CAD build for the part. Positions are in the model's coordinates, mm. Give positions to 0.01 mm unless a question says otherwise; leave off trailing zeros. Loops run counter-clockwise (first coordinate to the right, second up) from the corner with the lowest first, then second, coordinate; pieces in that order, holes last. Notation, with made-up numbers: M 42,-20 L 88,-20 A23 ccw 88,9 Z; hole C -27,-25.5 d1. An arc over 180 degrees is marked long. Answer as CSV lines item,"result".
```python
from build123d import *

# Parameters (mm, degrees)
EXTRUDE_1_DEPTH          = 2
CUT_EXTRUDE_1_DEPTH      = 2
PATTERN_START            = -2
PATTERN_LINEAR_1_DEPTH   = 2
PATTERN_CIRCULAR_2_COUNT = 5


# Read off the part's stored shape, not the designer's step: Линейный массив1
with BuildPart() as part:
    # Эскиз1 → Бобышка-Вытянуть1 (new body)
    with BuildSketch(Plane.XY):
        with BuildLine():
            Line((-21.160269083, 29.124611797), (0, 0))
            Line((0, 0), (21.160269083, 29.124611797))
            ThreePointArc((21.160269083, 29.124611797), (0, 36), (-21.160269083, 29.124611797))
        make_face()
    extrude_1 = extrude(amount=-EXTRUDE_1_DEPTH)

    # Эскиз3 → Вырез-Вытянуть1 (cut)
    with BuildSketch(Plane(origin=(0, 0, -2), x_dir=(-1, 0, 0), z_dir=(0, 0, -1))):
        with BuildLine():
            ThreePointArc((2.821419138, 8.689986144), (0, 9.136534635), (-2.821419138, 8.689986144))
            ThreePointArc((-2.821419138, 8.689986144), (-3.624317507, 7.115072112), (-2.049403475, 6.312173743))
            ThreePointArc((-2.049403475, 6.312173743), (0, 6.636534635), (2.049403475, 6.312173743))
            ThreePointArc((2.049403475, 6.312173743), (3.624317507, 7.115072112), (2.821419138, 8.689986144))
        make_face()
    cut_extrude_1 = extrude(amount=-CUT_EXTRUDE_1_DEPTH, mode=Mode.SUBTRACT)

    # Линейный массив1 outline → Линейный массив1 (cut)
    with BuildSketch(Plane.XY.offset(PATTERN_START)):
        with BuildLine():
            ThreePointArc((-5.868267845, 12.702937061), (-6.478815917, 11.043952114), (-4.81983097, 10.433404043))
            ThreePointArc((-4.81983097, 10.433404043), (0, 11.492897394), (4.81983097, 10.433404043))
            ThreePointArc((4.81983097, 10.433404043), (6.478815917, 11.043952114), (5.868267845, 12.702937061))
            ThreePointArc((5.868267845, 12.702937061), (0, 13.992897394), (-5.868267845, 12.702937061))
        make_face()
        with BuildLine():
            ThreePointArc((-14.786044108, 24.78794491), (-15.219207741, 23.074069399), (-13.50533223, 22.640905767))
            ThreePointArc((-13.50533223, 22.640905767), (0, 26.362940135), (13.50533223, 22.640905767))
            ThreePointArc((13.50533223, 22.640905767), (15.219207741, 23.074069399), (14.786044108, 24.78794491))
            ThreePointArc((14.786044108, 24.78794491), (0, 28.862940135), (-14.786044108, 24.78794491))
        make_face()
        with BuildLine():
            ThreePointArc((-17.738574213, 28.824927916), (-18.148018532, 27.10523162), (-16.428322236, 26.695787302))
            ThreePointArc((-16.428322236, 26.695787302), (0, 31.345730668), (16.428322236, 26.695787302))
            ThreePointArc((16.428322236, 26.695787302), (18.148018532, 27.10523162), (17.738574213, 28.824927916))
            ThreePointArc((17.738574213, 28.824927916), (0, 33.845730668), (-17.738574213, 28.824927916))
        make_face()
        with BuildLine():
            ThreePointArc((-8.858865357, 16.724555129), (-9.378370621, 15.034846787), (-7.688662279, 14.515341523))
            ThreePointArc((-7.688662279, 14.515341523), (0, 16.4259145), (7.688662279, 14.515341523))
            ThreePointArc((7.688662279, 14.515341523), (9.378370621, 15.034846787), (8.858865357, 16.724555129))
            ThreePointArc((8.858865357, 16.724555129), (0, 18.9259145), (-8.858865357, 16.724555129))
        make_face()
        with BuildLine():
            ThreePointArc((-11.827697591, 20.75389585), (-12.294790819, 19.04895482), (-10.589849789, 18.581861592))
            ThreePointArc((-10.589849789, 18.581861592), (0, 21.387624898), (10.589849789, 18.581861592))
            ThreePointArc((10.589849789, 18.581861592), (12.294790819, 19.04895482), (11.827697591, 20.75389585))
            ThreePointArc((11.827697591, 20.75389585), (0, 23.887624898), (-11.827697591, 20.75389585))
        make_face()
    pattern_linear_1 = extrude(amount=PATTERN_LINEAR_1_DEPTH, mode=Mode.SUBTRACT)

    # Круговой массив2: Бобышка-Вытянуть1, Вырез-Вытянуть1, Линейный массив1 ×5 about axis
    pattern_circular_2_axis = Axis((0, 0, 0), (0, 0, 1))
    add([extrude_1.rotate(pattern_circular_2_axis, i * 360 / PATTERN_CIRCULAR_2_COUNT) for i in range(1, PATTERN_CIRCULAR_2_COUNT)])
    add([cut_extrude_1.rotate(pattern_circular_2_axis, i * 360 / PATTERN_CIRCULAR_2_COUNT) for i in range(1, PATTERN_CIRCULAR_2_COUNT)], mode=Mode.SUBTRACT)
    add([pattern_linear_1.rotate(pattern_circular_2_axis, i * 360 / PATTERN_CIRCULAR_2_COUNT) for i in range(1, PATTERN_CIRCULAR_2_COUNT)], mode=Mode.SUBTRACT)


solid = part.part
```
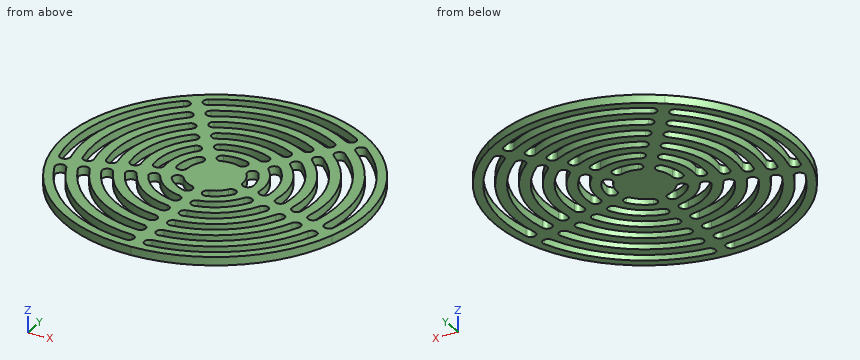
Q1. Cut at A-A (y = 28). Write the cut outline in (x, z), and give its area (3 significant figures).
Solution:
outline,"M -22.63,-2 L -18.31,-2 L -18.31,0 L -22.63,0 Z; M -14.09,-2 L -7,-2 L -7,0 L -14.09,0 Z; M 7,-2 L 14.09,-2 L 14.09,0 L 7,0 Z; M 18.31,-2 L 22.63,-2 L 22.63,0 L 18.31,0 Z"
area,"45.6 mm²"
Q2. Wall check: line 1 (Y direction, x = -22, z = -1.55); line 2 (Y direction, x = -19, z = -0.7); line 3 (Y direction, x = -29, z = -1.65). Give the ranges that are in metal, low to high. Write a range as [from, to].
Solution:
line 1,"y = [-28.5, -25.72], [-22.33, -18.68], [-14.53, -5.82], [9.31, 14.53], [18.68, 22.33], [25.72, 28.5]"
line 2,"y = [-30.58, -28.01], [-24.93, -21.73], [-18.28, -14.48], [-9.82, 9.82], [14.48, 18.28], [21.73, 30.58]"
line 3,"y = [-21.33, -17.45], [-11.9, 11.9], [17.45, 21.33]"
Q3. Cut at B-B (y = -27.5). Write the cut outline in (x, z), and give its area (3 significant figures).
Solution:
outline,"M -23.23,-2 L -19.73,-2 L -19.73,0 L -23.23,0 Z; M -15.04,-2 L -8.76,-2 L -8.76,0 L -15.04,0 Z; M -1.24,-2 L 1.24,-2 L 1.24,0 L -1.24,0 Z; M 8.76,-2 L 15.04,-2 L 15.04,0 L 8.76,0 Z; M 19.73,-2 L 23.23,-2 L 23.23,0 L 19.73,0 Z"
area,"44.1 mm²"
Q4. Cut at C-C (z = -0.4). Give the number of separate pieces and of enclosed holes in the cut face, and give its area (3 significant figures).
Solution:
separate pieces,"1"
enclosed holes,"30"
area,"2,400 mm²"
